```python
from build123d import *
from build123d.topology import SkipClean

# Parameters (mm, degrees)
SKETCH1_R           = 23.5
SKETCH1_R_2         = 15.05
BOSS_EXTRUDE1_DEPTH = 10
SKETCH2_R           = 23.5
SKETCH2_R_2         = 21
BOSS_EXTRUDE2_DEPTH = 5


with BuildPart() as part:
    # Sketch1 → Boss-Extrude1 (new, symmetric)
    with BuildSketch(Plane.XY):
        Circle(SKETCH1_R)
        Circle(SKETCH1_R_2, mode=Mode.SUBTRACT)
    extrude(amount=BOSS_EXTRUDE1_DEPTH, both=True)

    # Sketch2 → Boss-Extrude2 (add)
    with BuildSketch(Plane(origin=(0, 0, -10), x_dir=(-1, 0, 0), z_dir=(0, 0, -1))):
        Circle(SKETCH2_R)
        Circle(SKETCH2_R_2, mode=Mode.SUBTRACT)
    boss_extrude2 = extrude(amount=BOSS_EXTRUDE2_DEPTH)

    # Mirror1: Boss-Extrude2 across plane
    with SkipClean():  # the faces are left unmerged after this step: merging them gives an invalid solid
        add(boss_extrude2.mirror(Plane.XY))


solid = part.part
```
Work out the finished part from the listing and answer in its coordinate system (mm). A direction names the side the tool comes from. Round coordinates to 2 decimals unless told otherwise and drop trailing zeros. Write each loop counter-clockwise with the first axis right and the second up, starting at its lowest first coordinate (ties: lowest second). Pieces come first, ordered by that corner, then holes. Notation, with made-up numbers: (35.25, 78) - (55.25, 78) arc R31 ccw to (55.25, 109) - close; hole circle Ø10 at (-12, -22). An arc over 180 degrees is marked (long way). Return JSON: item names as keys, results as strings. Group by question number.
Q1. Find the intervals of material crossed by L1, parallel to Y at x = 0, z = -5.5; L2, parallel to Y at x = 0, z = -13.75; L3, parallel to X at y = -1, z = -9, in increasing order.
Q2. The part is cut by section D-D on y = -18.5. Write down the section's boundary in (x, z), then the cut area to 3 significant figures.
Q3. The part is cut by section C-C on z = -13. Write down the section's boundary in (x, y).
Q4. Each of these flat-tipped pins is pushed along its axis until it touches: pin 1 Ø6 at (y, z) = (17, -3.5) entering from +X; pin 2 Ø8 at (x, z) = (-10.5, 1) entering from +Y; pin 3 Ø4 at (y, z) = (13, 4) entering from -X. Where does it stop, or does it pass through?
Q5. The mould has two halves that part along X. Classify faces 1 (the cylindrical face through (-20.03, 6.31, 12.46)), 2 (the flat face through (18, -12, 15)): released by +X, released by -X, zero draft, split by the parting line, or undercut.
Q6. For faces 3 (the flat face through (9, -14, -10)), 4 (the flat face through (9, -14, 10)), 5 (the cylindrical face through (-3.263, -14.692, -0.14)), determine the directions among +Z, -Z, +X, -X, +Y, -Y from which every point of the face is accessible in a straight line to the end or side of a thin tool.
Q7. The part is cut by section A-A on y = 0. Write down the section's boundary in (x, z), then the cut area to 3 significant figures.
Solved:
{
 "1": {"L1": "-23.5 to -15.05, 15.05 to 23.5", "L2": "-23.5 to -21, 21 to 23.5", "L3": "-23.48 to -15.02, 15.02 to 23.48"},
 "2": {"outline": "(-14.49, -15) - (-9.94, -15) - (-9.94, -10) - (9.94, -10) - (9.94, -15) - (14.49, -15) - (14.49, 15) - (9.94, 15) - (9.94, 10) - (-9.94, 10) - (-9.94, 15) - (-14.49, 15) - close", "area": "671 mm²"},
 "3": {"outline": "circle Ø47 at (0, 0); hole circle Ø42 at (0, 0)"},
 "4": {"pin 1": "x = 18.87", "pin 2": "y = 22.58", "pin 3": "x = -20.77"},
 "5": {"face 1": "undercut", "face 2": "zero draft"},
 "6": {"face 3": "-Z", "face 4": "+Z", "face 5": "+Z, -Z"},
 "7": {"outline": "(-23.5, -15) - (-21, -15) - (-21, -10) - (-15.05, -10) - (-15.05, 10) - (-21, 10) - (-21, 15) - (-23.5, 15) - close; (15.05, -10) - (21, -10) - (21, -15) - (23.5, -15) - (23.5, 15) - (21, 15) - (21, 10) - (15.05, 10) - close", "area": "388 mm²"}
}
